The model under review builds one solid part; all positions refer to its coordinate system, in mm. A direction names the side the tool comes from. Coordinates: 2 decimals unless noted, no trailing zeros. Order: outer loops, then holes, each group sorted by start corner. A loop starts at its lowest first (then second) coordinate and runs counter-clockwise, first axis right, second up. Notation, with made-up numbers: M 24.25,53 L 39.25,53 A28 cw 39.25,90 Z; hole C 66,23.5 d10. An arc over 180 degrees is marked long. Write each question's results on one line, items separated by ' | '.
from build123d import *

# Parameters (mm, degrees)
F1_DEPTH  = 6
F2_W      = 2
F2_H      = 2
F3_DEPTH  = 5
F5_DEPTH  = 27
F7_DEPTH  = 3
F8_R      = 1.25
F9_DEPTH  = 3
F11_DEPTH = 4
F13_DEPTH = 3
F15_DEPTH = 3
F17_SIZE  = 0.99999
F18_SIZE  = 2


# Not quite as in the source:
# - a fillet or chamfer is up to 0.001 mm smaller than in the source, because OpenCascade refuses the exact size
# - a feature names something its author has since deleted; it is built from what else it names


with BuildPart() as f1:
    # F0 (on Top) → F1 (new body)
    with BuildSketch(Plane.XY):
        Polygon((-29.7051688433, 8.7922193985), (-30.7051688433, 8.7922193985), (-30.7051688433, -6.2077806015), (-15.7051688433, -6.2077806015), (-15.7051688433, -5.2077806015), (-15.7051688433, -0.2077806015), (-24.7051688433, -0.2077806015), (-24.7051688433, 8.7922193985), align=None)
    extrude(amount=F1_DEPTH)

    # F2 (on face) → F3 (join)
    with BuildSketch(Plane.XY.offset(6)):
        with Locations((-23.7051688433, -1.2077806015)):
            Rectangle(F2_W, F2_H)
        Polygon((-26.7051688433, -0.2077806015), (-30.7051688433, -0.2077806015), (-30.7051688433, -5.2077806015), (-29.7051688433, -6.2077806015), (-24.7051688433, -6.2077806015), (-24.7051688433, -2.2077806015), (-24.7051688433, -0.2077806015), align=None)
        with Locations((-25.7051688433, 0.7922193985)):
            Rectangle(F2_W, F2_H)
    extrude(amount=F3_DEPTH)

    # F4 (on face) → F5 (join)
    with BuildSketch(Plane.XY.offset(11)):
        Polygon((-26.7051688433, -6.2077806015), (-24.7051688433, -6.2077806015), (-24.7051688433, -2.2077806015), (-22.7051688433, -2.2077806015), (-22.7051688433, -0.2077806015), (-24.7051688433, -0.2077806015), (-24.7051688433, 1.7922193985), (-26.7051688433, 1.7922193985), (-26.7051688433, -0.2077806015), (-30.7051688433, -0.2077806015), (-30.7051688433, -2.2077806015), align=None)
    extrude(amount=F5_DEPTH)

    # F6 (on face) → F7 (join)
    with BuildSketch(Plane.XZ.offset(2.2077806015)):
        with BuildLine():
            ThreePointArc((-21.9412368208, 13), (-22.5076859202, 12.0704662693), (-22.7051688433, 11))
            ThreePointArc((-22.7051688433, 11), (-22.5076859202, 9.9295337307), (-21.9412368208, 9))
            ThreePointArc((-21.9412368208, 9), (-18.634702574, 8.1974829231), (-16.7051688433, 11))
            ThreePointArc((-16.7051688433, 11), (-18.634702574, 13.8025170769), (-21.9412368208, 13))
        make_face()
        with BuildLine():
            ThreePointArc((-18.4551688433, 11), (-19.7051688433, 9.75), (-20.9551688433, 11))
            ThreePointArc((-20.9551688433, 11), (-19.7051688433, 12.25), (-18.4551688433, 11))
        make_face(mode=Mode.SUBTRACT)
        with BuildLine():
            Line((-22.7051688433, 13), (-22.7051688433, 11))
            ThreePointArc((-22.7051688433, 11), (-22.5076859202, 12.0704662693), (-21.9412368208, 13))
            Line((-21.9412368208, 13), (-22.7051688433, 13))
        make_face()
        with BuildLine():
            Line((-22.7051688433, 11), (-22.7051688433, 9))
            Line((-22.7051688433, 9), (-21.9412368208, 9))
            ThreePointArc((-21.9412368208, 9), (-22.5076859202, 9.9295337307), (-22.7051688433, 11))
        make_face()
    extrude(amount=-F7_DEPTH)

    # F8 (on face) → F9 (join)
    with BuildSketch(Plane(origin=(-26.7051688433, 0, 0), x_dir=(0, -1, 0), z_dir=(-1, 0, 0))):
        with BuildLine():
            Line((-2.556151421, 9), (-1.7922193985, 9))
            Line((-1.7922193985, 9), (-1.7922193985, 11))
            ThreePointArc((-1.7922193985, 11), (-1.9897023217, 9.9295337307), (-2.556151421, 9))
        make_face()
        with BuildLine():
            ThreePointArc((-2.556151421, 13), (-1.9897023217, 12.0704662693), (-1.7922193985, 11))
            Line((-1.7922193985, 11), (-1.7922193985, 13))
            Line((-1.7922193985, 13), (-2.556151421, 13))
        make_face()
        with BuildLine():
            ThreePointArc((-2.556151421, 9), (-1.9897023217, 9.9295337307), (-1.7922193985, 11))
            ThreePointArc((-1.7922193985, 11), (-1.9897023217, 12.0704662693), (-2.556151421, 13))
            ThreePointArc((-2.556151421, 13), (-7.7922193985, 11), (-2.556151421, 9))
        make_face()
        with Locations((-4.7922193985, 11)):
            Circle(F8_R, mode=Mode.SUBTRACT)
    extrude(amount=-F9_DEPTH)

    # F10 (on face) → F11 (join)
    with BuildSketch(Plane.XY.offset(13)):
        Polygon((-22.7051688433, 0.7922193985), (-23.7051688433, 1.7922193985), (-24.7051688433, 1.7922193985), (-24.7051688433, -0.2077806015), (-22.7051688433, -0.2077806015), align=None)
    extrude(amount=-F11_DEPTH)

    # F12 (on face) → F13 (cut)
    with BuildSketch(Plane(origin=(0, 0, 0), x_dir=(1, 0, 0), z_dir=(0, 0, -1))):
        Polygon((-24.7051688433, -8.7922193985), (-24.7051688433, 0.2077806015), (-26.7051688433, -1.7922193985), (-26.7051688433, -8.7922193985), align=None)
        Polygon((-24.7051688433, 0.2077806015), (-15.7051688433, 0.2077806015), (-15.7051688433, 2.2077806015), (-22.7051688433, 2.2077806015), align=None)
    extrude(amount=-F13_DEPTH, mode=Mode.SUBTRACT)

    # F14 (on face) → F15 (join)
    with BuildSketch(Plane(origin=(0, 0, 3), x_dir=(1, 0, 0), z_dir=(0, 0, -1))):
        with BuildLine():
            Line((-16.7051688433, 0.2077806015), (-24.7051688433, 0.2077806015))
            Line((-24.7051688433, 0.2077806015), (-24.7051688433, -7.7922193985))
            Line((-24.7051688433, -7.7922193985), (-22.2863076734, -5.3733582286))
            ThreePointArc((-22.2863076734, -5.3733582286), (-21.4122756245, -3.0851126174), (-19.1240300132, -2.2110805685))
            Line((-19.1240300132, -2.2110805685), (-16.7051688433, 0.2077806015))
        make_face()
        with BuildLine():
            ThreePointArc((-19.1240300132, -2.2110805685), (-21.4122756245, -3.0851126174), (-22.2863076734, -5.3733582286))
            Line((-22.2863076734, -5.3733582286), (-20.7051688433, -3.7922193985))
            Line((-20.7051688433, -3.7922193985), (-19.1240300132, -2.2110805685))
        make_face()
        with BuildLine():
            Line((-20.7051688433, -3.7922193985), (-22.2863076734, -5.3733582286))
            ThreePointArc((-22.2863076734, -5.3733582286), (-19.2074603031, -8.2052708339), (-16.2909552809, -5.2064329609))
            ThreePointArc((-16.2909552809, -5.2064329609), (-17.1114168202, -3.1449742302), (-19.1240300132, -2.2110805685))
            Line((-19.1240300132, -2.2110805685), (-20.7051688433, -3.7922193985))
        make_face()
        with BuildLine():
            ThreePointArc((-18.0409552809, -5.2064329609), (-19.7693095714, -6.3612823766), (-20.1748387574, -4.3225494844))
            ThreePointArc((-20.1748387574, -4.3225494844), (-18.8126009904, -4.0515835453), (-18.0409552809, -5.2064329609))
        make_face(mode=Mode.SUBTRACT)
    extrude(amount=-F15_DEPTH)

    # F16: F1 across face


with BuildPart() as f1_1:
    add(f1.part)
    add(f1.part.mirror(Plane(origin=(-26.6681318062, -2.1707435644, 38), x_dir=(1, 0, 0), z_dir=(0, 0, 1))))

    # F17 (size 1 in the source; OpenCascade refuses exactly that, so slightly less here)
    f17_edges = [f1_1.edges().sort_by_distance(p)[0] for p in [
        (-24.705169, -6.207781, 38),
        (-20.205169, -6.207781, 6),
        (-30.705169, 4.292219, 6),
        (-30.705169, -0.207781, 38),
        (-30.705169, 4.292219, 70),
        (-20.205169, -6.207781, 70),
        (-15.705169, -6.207781, 73),
        (-30.705169, 8.792219, 73),
        (-23.205169, -6.207781, 76),
        (-30.705169, -6.207781, 73),
        (-30.705169, 1.292219, 76),
        (-30.705169, 8.792219, 3),
        (-30.705169, -6.207781, 3),
        (-15.705169, -6.207781, 3),
    ]]
    chamfer(f17_edges, length=F17_SIZE)

    # F18
    f18_edges = [f1_1.edges().sort_by_distance(p)[0] for p in [
        (-30.205169, -5.707781, 11),
        (-30.205169, -5.707781, 65),
    ]]
    chamfer(f18_edges, length=F18_SIZE)


solid = f1_1.part
1) Take a section at B-B on y = -3.5. State the section outline as (x, z) points, plus the area to 3 significant figures.
Solutions:
outline: M -30.71,0 L -15.71,0 L -15.71,6 L -24.71,6 L -24.71,70 L -15.71,70 L -15.71,76 L -29.71,76 L -30.71,75 L -30.71,65.79 L -29.58,65 L -29.41,65 L -29.41,11 L -29.58,11 L -30.71,10.21 Z | area: 493 mm2
2) For pin 1 (0.6 mm diameter, centred on x = -23.5, z = 7.5, fed in from +Y); pin 2 (3.5 mm diameter, centred on x = -23, y = 2, fed in from -Z); pin 3 (3.5 mm diameter, centred on y = 5, z = 1, fed in from +X); pin 4 (5 mm diameter, centred on x = -25, y = 0, fed in from -Z), all flat-tipped, find the tip position at first contact; note any pin that passes through.
Solutions:
pin 1: y = -0.21 | pin 2: z = 3 | pin 3: x = -26.71 | pin 4: z = 0
3) Take a section at A-A on z = 47. State the section outline as (x, y) points.
Solutions:
outline: M -30.71,-2.21 L -26.71,-6.21 L -25.71,-6.21 L -24.71,-5.21 L -24.71,-2.21 L -22.71,-2.21 L -22.71,-0.21 L -24.71,-0.21 L -24.71,1.79 L -26.71,1.79 L -26.71,-0.21 L -29.71,-0.21 L -30.71,-1.21 Z
4) To check wall thickness, follow line 1 along Z through (x, y) = (-22, -3.75); line 2 along Z through (x, y) = (-19, 3.5); line 3 along Y through (x, z) = (-29.5, 69.5). State the ranges of each line that lie inside material, in increasing order.
Solutions:
line 1: 0 to 6, 70 to 76 | line 2: 3 to 6, 70 to 73 | line 3: -6.21 to -0.21
5) The part is to be moulded in two halves that separate along Z. For faces 4 (the flat face through (-26, 1.792, 7)), 5 (the flat face through (-19, -2.208, 75)), 6 (the flat face through (-21, 3, 3)), say which applies: pulls with the +Z half, pulls with the -Z half, needs draft (parallel to the pull), parting line crosses it, or undercut.
Solutions:
face 4: undercut | face 5: needs draft | face 6: pulls with the -Z half
6) For faces 1 (the flat face through (-24, 1, 13)), 2 (the flat face through (-26.705, 1, 38)), 3 (the flat face through (-24.677, -0.236, 1.479)), list the 3-axis set-ups (+Z, -Z, +X, -X, +Y, -Y) from which the entire face can be reached by the end or side of a thin tool; tool diameter is ignored.
Solutions:
face 1: none | face 2: -X, +Y | face 3: -Z, +X, +Y
